Geometry: final body of the model. Coordinates: model frame, mm. A direction names the side the tool comes from. Round coordinates to 2 decimals unless told otherwise and drop trailing zeros. Write each loop counter-clockwise with the first axis right and the second up, starting at its lowest first coordinate (ties: lowest second). Pieces come first, ordered by that corner, then holes. Notation, with made-up numbers: M 32,44 L 64,44 A7 cw 64,54 Z; hole C 85,-8 d5. An arc over 180 degrees is marked long. Use one line per item in the form item = value. Start each with the question number.
Autodesk Inventor part; units mm, degrees
ref_plane "YZ Plane" through (0, 0, 0) normal (1, 0, 0) x (0, 1, 0)
ref_plane "XZ Plane" through (0, 0, 0) normal (0, 1, 0) x (-1, 0, 0)
ref_plane "XY Plane" through (0, 0, 0) normal (0, 0, 1) x (1, 0, 0)
sketch "Эскиз1" plane through (0, 0, 0) normal (0, 1, 0) x (-1, 0, 0)
  line L0 (0, 0) -> (0, -20)
  circle A0 centre (0, -20) radius 2
  line L1 (-3.5, 25) -> (3.5, 25)
  line L2 (3.5, 25) -> (3.5, -25)
  line L3 (3.5, -25) -> (-3.5, -25)
  line L4 (-3.5, -25) -> (-3.5, 25)
  line L5 (-3.5, 25) -> (3.5, -25) construction
  line L6 (3.5, 25) -> (-3.5, -25) construction
  line L7 (0, 0) -> (0, 20)
  circle A1 centre (0, 20) radius 2
  dimension "d0" = 20
  dimension "d1" = 4
  dimension "d2" = 7
  dimension "d3" = 50
  dimension "d4" = 20
  dimension "d5" = 4
extrude "Выдавливание1" add sketch "Эскиз1" along normal blind 4 contours A0 | L1 L2 L3 L4 | A1
sketch "Эскиз2" plane through (3.5, 0, 25) normal (1, 0, 0) x (0, 0, -1)
  line L0 (50, 0) -> (0, 0)
  line L1 (0, 4) -> (50, 4)
  line L2 (50, 4) -> (50, 0)
  line L3 (50, 0) -> (0, 0)
  line L4 (0, 0) -> (0, 4)
  point P0 (25, 0)
extrude "Выдавливание2" add sketch "Эскиз2" along normal blind 7
sketch "Эскиз3" plane through (0, 4, 0) normal (0, 1, 0) x (1, 0, 0)
  line L0 (-3.5, -25) -> (10.5, -25)
  line L1 (-3.5, 25) -> (10.5, 25)
  line L2 (10.5, -25) -> (3.5, -25)
  line L3 (3.5, -25) -> (3.5, 25)
  line L4 (3.5, 25) -> (10.5, 25)
  line L5 (10.5, 25) -> (10.5, -25)
  point P0 (0, 0)
  dimension "d10" = 7
extrude "Выдавливание3" add sketch "Эскиз3" along normal blind 30
sketch "Эскиз5" plane through (0, 4, 0) normal (0, 1, 0) x (1, 0, 0)
  line L0 (-7.5352, -8.6362) -> (-7.5352, -8.5162)
  arc A0 (-1.7352, -8.5162) -> (-7.5352, -8.5162) centre (-4.6352, -8.5162) ccw
  line L1 (-1.7352, -8.5162) -> (-1.7352, -8.6362)
  arc A1 (1.3648, -12.5541) -> (-1.7352, -8.6362) centre (-4.6352, -14.1162) ccw
  line L2 (1.3648, -12.5541) -> (1.3648, 1.4338)
  arc A2 (1.3648, 1.4338) -> (0.6148, 2.1838) centre (0.6148, 1.4338) ccw
  line L3 (0.6148, 2.1838) -> (-9.8852, 2.1838)
  arc A3 (-9.8852, 2.1838) -> (-10.6352, 1.4338) centre (-9.8852, 1.4338) ccw
  line L4 (-10.6352, 1.4338) -> (-10.6352, -12.5541)
  arc A4 (-7.5352, -8.6362) -> (-10.6352, -12.5541) centre (-4.6352, -14.1162) ccw
  line L5 (0.4648, -4.2162) -> (0.4648, 0.7838)
  arc A5 (-0.0352, -4.7162) -> (0.4648, -4.2162) centre (-0.0352, -4.2162) ccw
  line L6 (-9.2352, -4.7162) -> (-0.0352, -4.7162)
  arc A6 (-9.7352, -4.2162) -> (-9.2352, -4.7162) centre (-9.2352, -4.2162) ccw
  line L7 (-9.7352, 0.7838) -> (-9.7352, -4.2162)
  arc A7 (-9.2352, 1.2838) -> (-9.7352, 0.7838) centre (-9.2352, 0.7838) ccw
  line L8 (-0.0352, 1.2838) -> (-9.2352, 1.2838)
  arc A8 (0.4648, 0.7838) -> (-0.0352, 1.2838) centre (-0.0352, 0.7838) ccw
  arc A9 (-5.1852, 5.8865) -> (-4.0852, 5.8865) centre (-4.6352, 4.9338) ccw
  line L9 (-5.1852, 7.0838) -> (-5.1852, 5.8865)
  line L10 (-5.1852, 7.0838) -> (-9.8852, 7.0838)
  arc A10 (-9.8852, 7.0838) -> (-10.7352, 6.2338) centre (-9.8852, 6.2338) ccw
  line L11 (-10.7352, 6.2338) -> (-10.7352, 1.4338)
  arc A11 (-9.8852, 2.2838) -> (-10.7352, 1.4338) centre (-9.8852, 1.4338) ccw
  line L12 (0.6148, 2.2838) -> (-9.8852, 2.2838)
  arc A12 (1.4648, 1.4338) -> (0.6148, 2.2838) centre (0.6148, 1.4338) ccw
  line L13 (1.4648, 1.4338) -> (1.4648, 6.2338)
  arc A13 (1.4648, 6.2338) -> (0.6148, 7.0838) centre (0.6148, 6.2338) ccw
  line L14 (0.6148, 7.0838) -> (-4.0852, 7.0838)
  line L15 (-4.0852, 5.8865) -> (-4.0852, 7.0838)
  line L16 (-9.8852, -25.0162) -> (-5.1852, -25.0162)
  line L17 (-5.1852, -23.8188) -> (-5.1852, -25.0162)
  arc A14 (-4.0852, -23.8188) -> (-5.1852, -23.8188) centre (-4.6352, -22.8662) ccw
  line L18 (-4.0852, -25.0162) -> (-4.0852, -23.8188)
  line L19 (-4.0852, -25.0162) -> (0.6148, -25.0162)
  arc A15 (0.6148, -25.0162) -> (1.4648, -24.1662) centre (0.6148, -24.1662) ccw
  line L20 (1.4648, -24.1662) -> (1.4648, -19.3662)
  arc A16 (0.6148, -20.2162) -> (1.4648, -19.3662) centre (0.6148, -19.3662) ccw
  line L21 (-9.8852, -20.2162) -> (0.6148, -20.2162)
  arc A17 (-10.7352, -19.3662) -> (-9.8852, -20.2162) centre (-9.8852, -19.3662) ccw
  line L22 (-10.7352, -19.3662) -> (-10.7352, -24.1662)
  arc A18 (-10.7352, -24.1662) -> (-9.8852, -25.0162) centre (-9.8852, -24.1662) ccw
  line L23 (-10.7352, -19.3662) -> (-10.7352, -15.6782)
  line L24 (-10.7352, -12.5541) -> (-10.7352, -14.1162)
  line L25 (-10.7352, -14.1162) -> (-10.7352, -15.6782)
  line L26 (-10.7352, -12.5541) -> (-10.7352, 1.4338)
  line L27 (1.4648, 1.4338) -> (1.4648, -12.5541)
  line L28 (1.4648, -15.6782) -> (1.4648, -19.3662)
  line L29 (1.4648, -15.6782) -> (1.4648, -14.1162)
  line L30 (1.4648, -14.1162) -> (1.4648, -12.5541)
  arc A19 (-10.6352, -15.6782) -> (-6.1972, -20.1162) centre (-4.6352, -14.1162) ccw
  line L31 (-10.6352, -15.6782) -> (-10.6352, -19.3662)
  arc A20 (-10.6352, -19.3662) -> (-9.8852, -20.1162) centre (-9.8852, -19.3662) ccw
  line L32 (-9.8852, -20.1162) -> (-6.1972, -20.1162)
  line L33 (1.3648, -19.3662) -> (1.3648, -15.6782)
  arc A21 (-3.0731, -20.1162) -> (1.3648, -15.6782) centre (-4.6352, -14.1162) ccw
  line L34 (-3.0731, -20.1162) -> (0.6148, -20.1162)
  arc A22 (0.6148, -20.1162) -> (1.3648, -19.3662) centre (0.6148, -19.3662) ccw
  circle A23 centre (-4.6352, 4.9338) radius 1.1
  line L35 (-5.1852, 5.8865) -> (-5.1852, 7.0838)
  line L36 (-4.0852, 7.0838) -> (-5.1852, 7.0838)
  circle A24 centre (-4.6352, -22.8662) radius 1.1
  line L37 (-5.1852, -25.0162) -> (-5.1852, -23.8188)
  line L38 (-4.0852, -25.0162) -> (-5.1852, -25.0162)
  circle A25 centre (-4.6352, -14.1162) radius 0.8
  line L39 (-3.5, 25) -> (3.5, 25)
  line L40 (-13.5, 25) -> (-13.5, -25)
  line L41 (-13.5, -25) -> (-3.5, -25)
  line L42 (-3.5, -25) -> (-3.5, 25)
  point P0 (0, 0)
  point P1 (-4.6352, -8.9662)
  dimension "d16" = 10
extrude "Выдавливание5" cut sketch "Эскиз5" against normal blind 10 contours A4 L4 A3 L3 L42 L8 A7 L7 A6 L6 A0 L0 | L0 A0 L42 L21 A17 L23 L25 L24 L26 A11 L12 L3 A3 L4 A4 | L42 L6 A5 L5 A8 L8 L3 A2 L2 A1 L1 A0 | A0 L1 A1 L2 A2 L3 L42 L12 A12 L27 L30 L29 L28 A16 L21 | L42 L8 A8 L5 A5 L6 | L6 A6 L7 A7 L8 L42 | A19 L32 A20 L31 | A22 L34 A21 L33 | A25
move faces "Перенос1" translate (-6.504, 0, 0) faces at (-3.5, 2.6667, -9.8559) (-3.5, 1.3333, 23.4054)
sketch "Эскиз6" plane through (0, 4, 0) normal (0, 1, 0) x (1, 0, 0)
  arc A0 (1.4648, -18.6645) -> (1.4648, -9.5679) centre (-2.6, -14.1162) ccw
  line L0 (1.4648, -9.5679) -> (1.4648, -19.3662)
  point P0 (0, 0)
  point P1 (0.2532, -8.7246)
  point P2 (-5.4532, -8.7246)
extrude "Выдавливание6" cut sketch "Эскиз6" against normal blind 7
sketch "Эскиз7" plane through (0, 0, 0) normal (0, -1, 0) x (1, 0, 0)
  line L0 (-10.004, 25) -> (-10.004, 20.2162)
  line L1 (-10.004, 21.4561) -> (4.0826, 21.4561)
  line L2 (4.0826, 21.4561) -> (4.0826, -3.0396)
  line L3 (4.0826, -3.0396) -> (-10.004, -3.0396)
  line L4 (-10.004, -3.0396) -> (-10.004, 21.4561)
  point P0 (0, 0)
extrude "Выдавливание7" cut sketch "Эскиз7" against normal blind 0.3
sketch "Эскиз8" plane through (0, 4, 0) normal (0, 1, 0) x (1, 0, 0)
  line L0 (-7.5352, -8.6362) -> (-7.5352, -8.5162)
  arc A0 (-1.7352, -8.5162) -> (-7.5352, -8.5162) centre (-4.6352, -8.5162) ccw
  line L1 (-1.7352, -8.5162) -> (-1.7352, -8.6362)
  arc A1 (1.3648, -12.5541) -> (-1.7352, -8.6362) centre (-4.6352, -14.1162) ccw
  line L2 (1.3648, -12.5541) -> (1.3648, 1.4338)
  arc A2 (1.3648, 1.4338) -> (0.6148, 2.1838) centre (0.6148, 1.4338) ccw
  line L3 (0.6148, 2.1838) -> (-9.8852, 2.1838)
  arc A3 (-9.8852, 2.1838) -> (-10.6352, 1.4338) centre (-9.8852, 1.4338) ccw
  line L4 (-10.6352, 1.4338) -> (-10.6352, -12.5541)
  arc A4 (-7.5352, -8.6362) -> (-10.6352, -12.5541) centre (-4.6352, -14.1162) ccw
  line L5 (0.4648, -4.2162) -> (0.4648, 0.7838)
  arc A5 (-0.0352, -4.7162) -> (0.4648, -4.2162) centre (-0.0352, -4.2162) ccw
  line L6 (-9.2352, -4.7162) -> (-0.0352, -4.7162)
  arc A6 (-9.7352, -4.2162) -> (-9.2352, -4.7162) centre (-9.2352, -4.2162) ccw
  line L7 (-9.7352, 0.7838) -> (-9.7352, -4.2162)
  arc A7 (-9.2352, 1.2838) -> (-9.7352, 0.7838) centre (-9.2352, 0.7838) ccw
  line L8 (-0.0352, 1.2838) -> (-9.2352, 1.2838)
  arc A8 (0.4648, 0.7838) -> (-0.0352, 1.2838) centre (-0.0352, 0.7838) ccw
  arc A9 (-5.1852, 5.8865) -> (-4.0852, 5.8865) centre (-4.6352, 4.9338) ccw
  line L9 (-5.1852, 7.0838) -> (-5.1852, 5.8865)
  line L10 (-5.1852, 7.0838) -> (-9.8852, 7.0838)
  arc A10 (-9.8852, 7.0838) -> (-10.7352, 6.2338) centre (-9.8852, 6.2338) ccw
  line L11 (-10.7352, 6.2338) -> (-10.7352, 1.4338)
  arc A11 (-9.8852, 2.2838) -> (-10.7352, 1.4338) centre (-9.8852, 1.4338) ccw
  line L12 (0.6148, 2.2838) -> (-9.8852, 2.2838)
  arc A12 (1.4648, 1.4338) -> (0.6148, 2.2838) centre (0.6148, 1.4338) ccw
  line L13 (1.4648, 1.4338) -> (1.4648, 6.2338)
  arc A13 (1.4648, 6.2338) -> (0.6148, 7.0838) centre (0.6148, 6.2338) ccw
  line L14 (0.6148, 7.0838) -> (-4.0852, 7.0838)
  line L15 (-4.0852, 5.8865) -> (-4.0852, 7.0838)
  line L16 (-9.8852, -25.0162) -> (-5.1852, -25.0162)
  line L17 (-5.1852, -23.8188) -> (-5.1852, -25.0162)
  arc A14 (-4.0852, -23.8188) -> (-5.1852, -23.8188) centre (-4.6352, -22.8662) ccw
  line L18 (-4.0852, -25.0162) -> (-4.0852, -23.8188)
  line L19 (-4.0852, -25.0162) -> (0.6148, -25.0162)
  arc A15 (0.6148, -25.0162) -> (1.4648, -24.1662) centre (0.6148, -24.1662) ccw
  line L20 (1.4648, -24.1662) -> (1.4648, -19.3662)
  arc A16 (0.6148, -20.2162) -> (1.4648, -19.3662) centre (0.6148, -19.3662) ccw
  line L21 (-9.8852, -20.2162) -> (0.6148, -20.2162)
  arc A17 (-10.7352, -19.3662) -> (-9.8852, -20.2162) centre (-9.8852, -19.3662) ccw
  line L22 (-10.7352, -19.3662) -> (-10.7352, -24.1662)
  arc A18 (-10.7352, -24.1662) -> (-9.8852, -25.0162) centre (-9.8852, -24.1662) ccw
  line L23 (-10.7352, -19.3662) -> (-10.7352, -15.6782)
  line L24 (-10.7352, -12.5541) -> (-10.7352, -14.1162)
  line L25 (-10.7352, -14.1162) -> (-10.7352, -15.6782)
  line L26 (-10.7352, -12.5541) -> (-10.7352, 1.4338)
  line L27 (1.4648, 1.4338) -> (1.4648, -12.5541)
  line L28 (1.4648, -15.6782) -> (1.4648, -19.3662)
  line L29 (1.4648, -15.6782) -> (1.4648, -14.1162)
  line L30 (1.4648, -14.1162) -> (1.4648, -12.5541)
  arc A19 (-10.6352, -15.6782) -> (-6.1972, -20.1162) centre (-4.6352, -14.1162) ccw
  line L31 (-10.6352, -15.6782) -> (-10.6352, -19.3662)
  arc A20 (-10.6352, -19.3662) -> (-9.8852, -20.1162) centre (-9.8852, -19.3662) ccw
  line L32 (-9.8852, -20.1162) -> (-6.1972, -20.1162)
  line L33 (1.3648, -19.3662) -> (1.3648, -15.6782)
  arc A21 (-3.0731, -20.1162) -> (1.3648, -15.6782) centre (-4.6352, -14.1162) ccw
  line L34 (-3.0731, -20.1162) -> (0.6148, -20.1162)
  arc A22 (0.6148, -20.1162) -> (1.3648, -19.3662) centre (0.6148, -19.3662) ccw
  circle A23 centre (-4.6352, 4.9338) radius 1.1
  line L35 (-5.1852, 5.8865) -> (-5.1852, 7.0838)
  line L36 (-4.0852, 7.0838) -> (-5.1852, 7.0838)
  circle A24 centre (-4.6352, -22.8662) radius 1.1
  line L37 (-5.1852, -25.0162) -> (-5.1852, -23.8188)
  line L38 (-4.0852, -25.0162) -> (-5.1852, -25.0162)
  circle A25 centre (-4.6352, -14.1162) radius 0.8
  line L39 (-3.5, 25) -> (3.5, 25)
  line L40 (-13.5, 25) -> (-13.5, -25)
  line L41 (-13.5, -25) -> (-3.5, -25)
  line L42 (-3.5, -25) -> (-3.5, 25)
  point P0 (0, 0)
  point P1 (0, 0)
  point P2 (-4.6352, -8.9662)
  dimension "d26" = 10
extrude "Выдавливание8" cut sketch "Эскиз8" against normal through all contours A24 A14 | A9 A23
move faces "Перенос2" translate (-2.5, 0, 0) faces at (10.5, 11.3333, -8.3333)
chamfer "Фаска1" distance 2 angle 45 2 edges at (3.5, 19, 25) (3.5, 19, -25)
chamfer "Фаска2" distance 2 angle 45 1 edges at (3.5, 19, 23)
properties part number "000.705 - Пассивный прижим"
1. Ray query, probe 1 along X at (y, z) = (9.5, 5); probe 2 along Y at (x, z) = (-9, -6.5); probe 3 along Z at (x, y) = (-6, 3). Return the intervals inside material, ascending.
2. Section query A-A (x = -6.5). Return loops of the section in (y, z), then the cut area to 3 significant figures.
3. Set-up query: faces 4 (the face through (4.5, 18.8, -24)), 5 (the face through (2, 0.3, 8)), 6 (the face through (4.217, 19.21, 22.731)), 7 (the face through (-4.643, 2.028, 23.966)), 8 (the face through (1.465, 2, 4)). Return all of +Z, -Z, +X, -X, +Y, -Y with unobstructed straight access to the full face (end or side cutting, diameter ignored); none if empty.
4. Section query D-D (x = 2). Return loops of the section in (y, z), then the cut area to 3 significant figures.
5. Section query C-C (z = 8.5). Return loops of the section in (x, y), then the cut area to 3 significant figures.
6. Section query B-B (y = 23). Return loops of the section in (x, z), then the cut area to 3 significant figures.
7. Pull-direction query (X, two-part tool) for faces 1 (the face through (-4.627, 2.028, -6.034)), 2 (the face through (3.5, 19, -1)), 3 (the face through (1, 0, -6)); classes: released by +X, released by -X, zero draft, split by the parting line, or undercut.
8. Contact query for flat-ended pins moving along their axis: pin 1 (5.5 mm diameter, centred on x = -2, z = 21.5, fed in from +Y); pin 2 (15 mm diameter, centred on y = 14.5, z = 0.5, fed in from -X); pin 3 (1.8 mm diameter, centred on y = 2.5, z = 2.5, fed in from -X). Output: stop coordinate, or through.
Checks:
q1.probe_1 = 3.5 to 8
q1.probe_2 = 0 to 4
q1.probe_3 = -25 to -2.28, 20.22 to 25
q2.outline = M 0,-25 L 4,-25 L 4,-2.28 L 0.3,-2.28 L 0.3,-3.04 L 0,-3.04 Z; M 0,21.46 L 0.3,21.46 L 0.3,20.22 L 4,20.22 L 4,25 L 0,25 Z
q2.area = 109 mm^2
q3.face_4 = -Z, -X, +Y
q3.face_5 = -X, -Y
q3.face_6 = +Z, -X, +Y
q3.face_7 = +Y, -Y
q3.face_8 = -X, +Y, -Y
q4.outline = M 0,-25 L 4,-25 L 4,10.11 L 0.3,10.11 L 0.3,-3.04 L 0,-3.04 Z; M 0,21.46 L 0.3,21.46 L 0.3,18.12 L 4,18.12 L 4,25 L 0,25 Z
q4.area = 163 mm^2
q5.outline = M 1.46,0.3 L 4.08,0.3 L 4.08,0 L 8,0 L 8,34 L 3.5,34 L 3.5,4 L 1.46,4 Z
q5.area = 160 mm^2
q6.outline = M 3.5,-23 L 5.5,-25 L 8,-25 L 8,25 L 5.5,25 L 4.91,24.41 L 3.5,21 Z
q6.area = 220 mm^2
q7.face_1 = undercut
q7.face_2 = released by -X
q7.face_3 = zero draft
q8.pin_1 = 4
q8.pin_2 = 3.5
q8.pin_3 = 1.46
